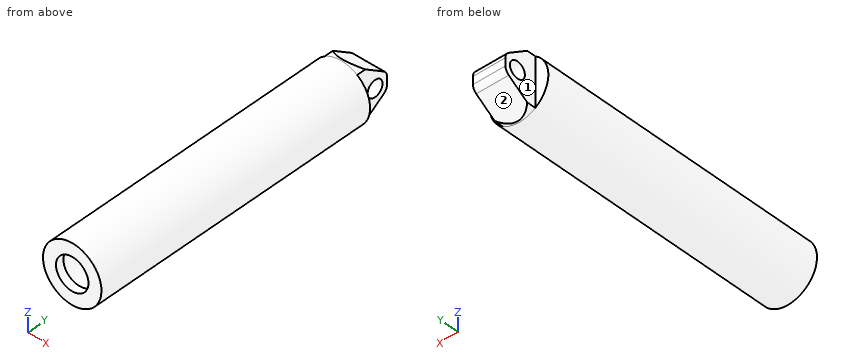
from build123d import *
from build123d.topology import SkipClean

# Parameters (mm, degrees)
CROQUIS1_R                   = 18
SALIENTE_EXTRUIR1_DEPTH      = 180
VACIADO1_T                   = -1
CROQUIS3_R                   = 17
CROQUIS3_R_2                 = 10
SALIENTE_EXTRUIR2_DEPTH      = 5
SALIENTE_EXTRUIR3_DEPTH      = 10
SALIENTE_EXTRUIR3_DEPTH_BACK = 10
CROQUIS4_R                   = 5
CORTAR_EXTRUIR1_DEPTH        = 37


with BuildPart() as part:
    # Croquis1 → Saliente-Extruir1 (new body)
    with BuildSketch(Plane(origin=(0, 0, 0), x_dir=(1, 0, 0), z_dir=(0, 1, 0))):
        with Locations(Location((0, 0, 0), (0, 0, 90))):
            Circle(CROQUIS1_R)
    extrude(amount=SALIENTE_EXTRUIR1_DEPTH)

    # Vaciado1
    vaciado1_openings = [part.faces().sort_by_distance(p)[0] for p in [
        (0, 0, 0),
    ]]
    offset(amount=VACIADO1_T, openings=vaciado1_openings, kind=Kind.INTERSECTION)

    # Croquis3 → Saliente-Extruir2 (add)
    with BuildSketch(Plane.XZ):
        with Locations(Location((0, 0, 0), (0, 0, 270))):
            Circle(CROQUIS3_R)
        with Locations(Location((0, 0, 0), (0, 0, 270))):
            Circle(CROQUIS3_R_2, mode=Mode.SUBTRACT)
    extrude(amount=-SALIENTE_EXTRUIR2_DEPTH)

    # Croquis4 → Saliente-Extruir3 (add, two sides: drawn at the far end of the back side and taken through both)
    with BuildSketch(Plane(origin=(0, 0, 0), x_dir=(0, 0, -1), z_dir=(1, 0, 0)).offset(-SALIENTE_EXTRUIR3_DEPTH_BACK)):
        with BuildLine():
            Line((-2.367587924, 200), (2.367587924, 200))
            ThreePointArc((2.367587924, 200), (4.696897355, 199.424287239), (6.489801521, 197.82972703))
            Line((6.489801521, 197.82972703), (18.729162566, 180))
            Line((18.729162566, 180), (-18.729162566, 180))
            Line((-18.729162566, 180), (-6.489801521, 197.82972703))
            ThreePointArc((-6.489801521, 197.82972703), (-4.696897355, 199.424287239), (-2.367587924, 200))
        make_face()
        with Locations((0, 192)):
            Circle(CROQUIS4_R, mode=Mode.SUBTRACT)
    extrude(amount=SALIENTE_EXTRUIR3_DEPTH + SALIENTE_EXTRUIR3_DEPTH_BACK)

    # Croquis5 → Cortar-Extruir1 (cut)
    with SkipClean():  # the faces are left unmerged after this step: merging them gives an invalid solid
        with BuildSketch(Plane(origin=(0, 180, 0), x_dir=(1, 0, 0), z_dir=(0, 1, 0))):
            with BuildLine():
                Line((34.507590677, -30.013991489), (34.507590677, -14.966629547))
                Line((34.507590677, -14.966629547), (10, -14.966629547))
                ThreePointArc((10, -14.966629547), (-18, 0), (10, 14.966629547))
                Line((10, 14.966629547), (10, 20.876886583))
                Line((10, 20.876886583), (-23.183234279, 20.876886583))
                Line((-23.183234279, 20.876886583), (-23.183234279, -30.013991489))
                Line((-23.183234279, -30.013991489), (34.507590677, -30.013991489))
            make_face()
        extrude(amount=CORTAR_EXTRUIR1_DEPTH, mode=Mode.SUBTRACT)


solid = part.part
The model under review builds one solid part; all positions refer to its coordinate system, in mm. Face numbers are marked on the shaded views. A direction names the side the tool comes from. Round coordinates to 2 decimals unless told otherwise and drop trailing zeros. Loops run counter-clockwise (first coordinate to the right, second up) from the corner with the lowest first, then second, coordinate; pieces in that order, holes last. Notation, with made-up numbers: (3.25, -28.75) -> (40.25, -28.75) arc R15 ccw to (40.25, -13.75) -> close; hole circle Ø8 at (12, 30.5). An arc over 180 degrees is marked (long way). One line per question, with ' | ' between items. Start each with the question number.
Item 1: Add section A-A, the plane x = 0. Write out the cut boundary in (y, z).
Item 2: For pin 1 (4 mm diameter, centred on x = 8, y = 47.5, fed in from +Z); pin 2 (6.5 mm diameter, centred on x = -15, z = 4.5, fed in from +Y); pin 3 (4 mm diameter, centred on y = 129.5, z = -6.5, fed in from -X), all flat-tipped, find the tip position at first contact; note any pin that passes through.
Item 3: Add section D-D, the plane x = 15. Write out the cut boundary in (y, z), then the cut area to 3 significant figures.
Item 4: Wall thickness on line 1 along X through (y, z) = (108, 0); line 2 along Y through (x, z) = (-12, -11.5); line 3 along Y through (x, z) = (4.25, 0): over which ranges is each line inside the solid? List them lowest first. Write a range as [from, to].
Item 5: Add section B-B, the plane z = 0. Write out the cut boundary in (x, y), then the cut area to 3 significant figures.
Item 6: Add section C-C, the plane y = 60. Write out the cut boundary in (x, z).
Item 7: Machinability: for the marked faces 1 and 2, which of the approach directions +Z, -Z, +X, -X, +Y, -Y give a long, thin tool a straight path to every point of the face, cutting with its end or side? Answer none if there is none.
Return value:
1) outline: (0, -18) -> (181.06, -18) -> (197.83, -6.49) arc R5 ccw to (200, -2.37) -> (200, 2.37) arc R5 ccw to (197.83, 6.49) -> (181.06, 18) -> (0, 18) -> (0, 10) -> (5, 10) -> (5, 17) -> (179, 17) -> (179, -17) -> (5, -17) -> (5, -10) -> (0, -10) -> close; hole circle Ø10 at (192, 0)
2) pin 1: stops at z = 16.97 | pin 2: stops at y = 180 | pin 3: stops at x = -17.43
3) outline: (0, -9.95) -> (180, -9.95) -> (180, 9.95) -> (0, 9.95) -> close; hole (5, -8) -> (179, -8) -> (179, 8) -> (5, 8) -> close | area: 798 mm2
4) line 1: x = [-18, -17], [17, 18] | line 2: y = [0, 5], [179, 180] | line 3: y = [179, 187], [197, 200]
5) outline: (-18, 0) -> (-10, 0) -> (-10, 5) -> (-17, 5) -> (-17, 179) -> (17, 179) -> (17, 5) -> (10, 5) -> (10, 0) -> (18, 0) -> (18, 180) -> (10, 180) -> (10, 187) -> (-10, 187) -> (-10, 180) -> (-18, 180) -> close; (-10, 197) -> (10, 197) -> (10, 200) -> (-10, 200) -> close | area: 664 mm2
6) outline: circle Ø36 at (0, 0); hole circle Ø34 at (0, 0)
7) face 1: +Z, -Z, -X, +Y | face 2: -Z, +X, -X, +Y
